The listing builds one solid part. Answer for the finished solid, in the listing's coordinates (mm). Face numbers are marked on the shaded views. A direction names the side the tool comes from. Coordinates: 2 decimals unless noted, no trailing zeros. Order: outer loops, then holes, each group sorted by start corner. A loop starts at its lowest first (then second) coordinate and runs counter-clockwise, first axis right, second up. Notation, with made-up numbers: (35, 11.5) -> (51, 11.5) arc R19 cw to (51, 38.5) -> close; hole circle Ø11 at (15.25, 77.5). An arc over 180 degrees is marked (long way). Answer in a Markdown table with one row per item. Add a question column.
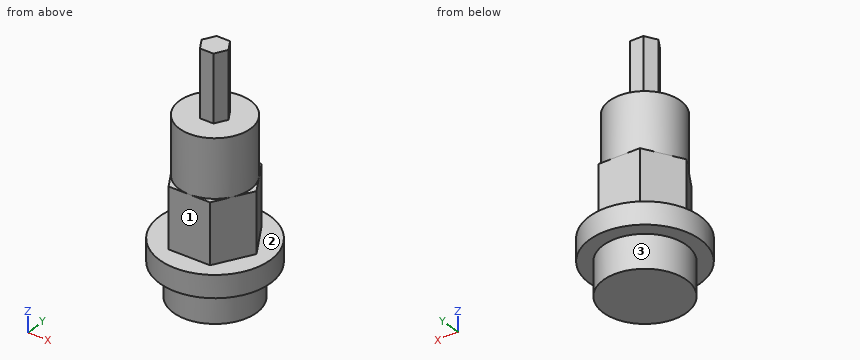
```python
from build123d import *

# Parameters (mm, degrees)
SKETCH1_R           = 3.75
BOSS_EXTRUDE1_DEPTH = 3
SKETCH2_R           = 5
BOSS_EXTRUDE2_DEPTH = 2
BOSS_EXTRUDE3_DEPTH = 5.4
SKETCH4_R           = 3.204293994
BOSS_EXTRUDE4_DEPTH = 5.2
BOSS_EXTRUDE5_DEPTH = 6


with BuildPart() as part:
    # Sketch1 → Boss-Extrude1 (new body)
    with BuildSketch(Plane.XY):
        Circle(SKETCH1_R)
    extrude(amount=BOSS_EXTRUDE1_DEPTH)

    # Sketch2 → Boss-Extrude2 (add)
    with BuildSketch(Plane.XY.offset(3)):
        Circle(SKETCH2_R)
    extrude(amount=BOSS_EXTRUDE2_DEPTH)

    # Sketch3 → Boss-Extrude3 (add)
    with BuildSketch(Plane.XY.offset(5)):
        Polygon((3.7, 0), (1.85, 3.204293994), (-1.85, 3.204293994), (-3.7, 0), (-1.85, -3.204293994), (1.85, -3.204293994), align=None)
    extrude(amount=BOSS_EXTRUDE3_DEPTH)

    # Sketch4 → Boss-Extrude4 (add)
    with BuildSketch(Plane.XY.offset(10.4)):
        Circle(SKETCH4_R)
    extrude(amount=BOSS_EXTRUDE4_DEPTH)

    # Sketch5 → Boss-Extrude5 (add)
    with BuildSketch(Plane.XY.offset(15.6)):
        Polygon((1.2, 0), (0.6, 1.039230485), (-0.6, 1.039230485), (-1.2, 0), (-0.6, -1.039230485), (0.6, -1.039230485), align=None)
    extrude(amount=BOSS_EXTRUDE5_DEPTH)


solid = part.part
```
Q1. Given pin 1 (1.8 mm diameter, centred on x = -0.5, y = -2.5, fed in from +Z); pin 2 (3 mm diameter, centred on x = 0.5, z = 9, fed in from +Y); pin 3 (6 mm diameter, centred on x = -4, z = 3.5, fed in from -Y), each flat-ended and moving along its own axis, determine where each tip first touches the part or whether it passes through.
Q2. For the marked faces 1, 2 and 3, determine the directions among +Z, -Z, +X, -X, +Y, -Y from which every point of the face is accessible in a straight line to the end or side of a thin tool.
Q3. A cutting plane is placed at D-D (y = -0.25). Determine the outline of the cut face in (x, z), then the cut area to 3 significant figures.
Q4. Straight lines are drawn through the part: line 1 (Z direction, x = -4.25, y = 2.5); line 2 (Y direction, x = 0, z = 9.75); line 3 (Z direction, x = -2.5, y = 1.5). For each, find the intervals that lie inside material, in ascending order.
Q5. A cutting plane is placed at C-C (x = 1.5). Determine the outline of the cut face in (y, z), then the cut area to 3 significant figures.
Q6. A cutting plane is placed at A-A (z = 5.5). Determine the outline of the cut face in (x, y), then the cut area to 3 significant figures.
Q7. A cutting plane is placed at B-B (y = 2.75). Determine the outline of the cut face in (x, z), then the cut area to 3 significant figures.
Returned:
| question | item | result |
|---|---|---|
| 1 | pin 1 | stops at z = 15.6 |
| 1 | pin 2 | stops at y = 3.2 |
| 1 | pin 3 | stops at y = -4.9 |
| 2 | face 1 | +Z, +X, -X, -Y |
| 2 | face 2 | +Z |
| 2 | face 3 | -Z |
| 3 | outline | (-4.99, 3) -> (-3.74, 3) -> (-3.74, 0) -> (3.74, 0) -> (3.74, 3) -> (4.99, 3) -> (4.99, 5) -> (3.56, 5) -> (3.56, 10.4) -> (3.19, 10.4) -> (3.19, 15.6) -> (1.06, 15.6) -> (1.06, 21.6) -> (-1.06, 21.6) -> (-1.06, 15.6) -> (-3.19, 15.6) -> (-3.19, 10.4) -> (-3.56, 10.4) -> (-3.56, 5) -> (-4.99, 5) -> close |
| 3 | area | 127 mm² |
| 4 | line 1 | z = 3 to 5 |
| 4 | line 2 | y = -3.2 to 3.2 |
| 4 | line 3 | z = 0 to 15.6 |
| 5 | outline | (-4.77, 3) -> (-3.44, 3) -> (-3.44, 0) -> (3.44, 0) -> (3.44, 3) -> (4.77, 3) -> (4.77, 5) -> (3.2, 5) -> (3.2, 10.4) -> (2.83, 10.4) -> (2.83, 15.6) -> (-2.83, 15.6) -> (-2.83, 10.4) -> (-3.2, 10.4) -> (-3.2, 5) -> (-4.77, 5) -> close |
| 5 | area | 104 mm² |
| 6 | outline | (-3.7, 0) -> (-1.85, -3.2) -> (1.85, -3.2) -> (3.7, 0) -> (1.85, 3.2) -> (-1.85, 3.2) -> close |
| 6 | area | 35.6 mm² |
| 7 | outline | (-4.18, 3) -> (-2.55, 3) -> (-2.55, 0) -> (2.55, 0) -> (2.55, 3) -> (4.18, 3) -> (4.18, 5) -> (2.11, 5) -> (2.11, 10.4) -> (1.64, 10.4) -> (1.64, 15.6) -> (-1.64, 15.6) -> (-1.64, 10.4) -> (-2.11, 10.4) -> (-2.11, 5) -> (-4.18, 5) -> close |
| 7 | area | 71.9 mm² |
